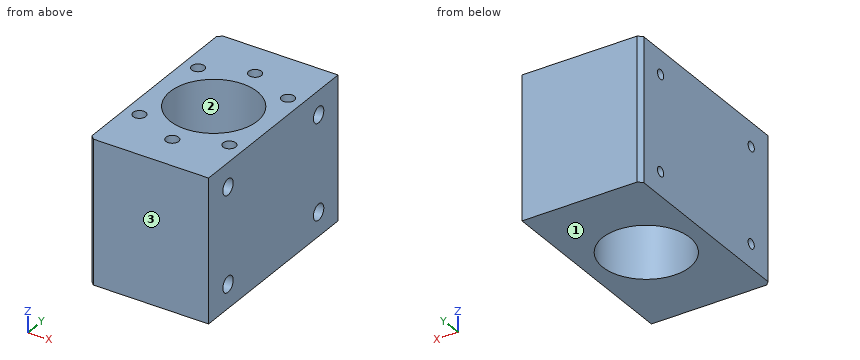
```python
from build123d import *

# Parameters (mm, degrees)
SKETCH_4_R          = 11
EXTRUDE_2_DEPTH     = 36
SKETCH_5_R          = 1.6
CUT_EXTRUDE_2_DEPTH = 10
SKETCH_6_R          = 2
CUT_EXTRUDE_3_DEPTH = 10
SKETCH_9_R          = 1.2
CUT_EXTRUDE_5_DEPTH = 5


with BuildPart() as part:
    # 草图4 → 凸台-拉伸2 (new body)
    with BuildSketch(Plane.XY):
        Polygon((15, 25), (-14, 25), (-15, 24), (-15, -24), (-14, -25), (15, -25), align=None)
        Circle(SKETCH_4_R, mode=Mode.SUBTRACT)
    extrude(amount=EXTRUDE_2_DEPTH)

    # 草图5 → 切除-拉伸2 (cut)
    with BuildSketch(Plane.XY.offset(36)):
        with Locations((0, 16)):
            Circle(SKETCH_5_R)
        with Locations((11.313708499, 11.313708499)):
            Circle(SKETCH_5_R)
        with Locations((11.313708499, -11.313708499)):
            Circle(SKETCH_5_R)
        with Locations((0, -16)):
            Circle(SKETCH_5_R)
        with Locations((-11.313708499, -11.313708499)):
            Circle(SKETCH_5_R)
        with Locations((-11.313708499, 11.313708499)):
            Circle(SKETCH_5_R)
    extrude(amount=-CUT_EXTRUDE_2_DEPTH, mode=Mode.SUBTRACT)

    # 草图6 → 切除-拉伸3 (cut)
    with BuildSketch(Plane(origin=(15, 0, 0), x_dir=(0, 0, -1), z_dir=(1, 0, 0))):
        with Locations((-6, 17.5)):
            Circle(SKETCH_6_R)
        with Locations((-30, 17.5)):
            Circle(SKETCH_6_R)
        with Locations((-30, -17.5)):
            Circle(SKETCH_6_R)
        with Locations((-6, -17.5)):
            Circle(SKETCH_6_R)
    extrude(amount=-CUT_EXTRUDE_3_DEPTH, mode=Mode.SUBTRACT)

    # 草图9 → 切除-拉伸5 (cut)
    with BuildSketch(Plane.ZY.offset(15)):
        with Locations((6, 17.5)):
            Circle(SKETCH_9_R)
        with Locations((30, 17.5)):
            Circle(SKETCH_9_R)
        with Locations((6, -17.5)):
            Circle(SKETCH_9_R)
        with Locations((30, -17.5)):
            Circle(SKETCH_9_R)
    extrude(amount=-CUT_EXTRUDE_5_DEPTH, mode=Mode.SUBTRACT)


solid = part.part
```
Input: part model. Units: mm. Frame: model coordinates. Face numbers are marked on the shaded views. Give positions to 0.01 mm unless a question says otherwise; leave off trailing zeros. Loops run counter-clockwise (first coordinate to the right, second up) from the corner with the lowest first, then second, coordinate; pieces in that order, holes last.
1) Line query: L1, parallel to Y at x = 13, z = 30; L2, parallel to Y at x = -12.9, z = 6; L3, parallel to Y at x = 0, z = 29.5. Output: solid intervals per line, ascending.
A:
L1: y = -25 to -19.5, -15.5 to 15.5, 19.5 to 25
L2: y = -25 to -18.7, -16.3 to 16.3, 18.7 to 25
L3: y = -25 to -17.6, -14.4 to -11, 11 to 14.4, 17.6 to 25
2) Mould query, pull axis Y, two halves, no side actions, for the marked faces 1, 2 and 3. Classes: released by +Y, released by -Y, zero draft, split by the parting line, or undercut.
A:
face 1: zero draft
face 2: undercut
face 3: released by -Y
3) Section query D-D on z = 6. Return the cut outline in (x, y), and give its area (3 significant figures).
A:
outline: (-15, -24) - (-14, -25) - (15, -25) - (15, -19.5) - (5, -19.5) - (5, -15.5) - (15, -15.5) - (15, 15.5) - (5, 15.5) - (5, 19.5) - (15, 19.5) - (15, 25) - (-14, 25) - (-15, 24) - (-15, 18.7) - (-10, 18.7) - (-10, 16.3) - (-15, 16.3) - (-15, -16.3) - (-10, -16.3) - (-10, -18.7) - (-15, -18.7) - close; hole circle Ø22 at (0, 0)
area: 1,010 mm2
4) Section query A-A on y = 0. Return the cut outline in (x, z), and give its area (3 significant figures).
A:
outline: (-15, 0) - (-11, 0) - (-11, 36) - (-15, 36) - close; (11, 0) - (15, 0) - (15, 36) - (11, 36) - close
area: 288 mm2
5) Section query B-B on z = 13. Return the cut outline in (x, y), and give its area (3 significant figures).
A:
outline: (-15, -24) - (-14, -25) - (15, -25) - (15, 25) - (-14, 25) - (-15, 24) - close; hole circle Ø22 at (0, 0)
area: 1,120 mm2
6) Contact query for flat-ended pins moving along their axis: pin 1 (1.9 mm diameter, centred on x = -11.31, y = -11.31, fed in from +Z); pin 2 (1.9 mm diameter, centred on y = -17.5, z = 6, fed in from -X); pin 3 (13 mm diameter, centred on x = 0, y = 0, fed in from -Z); pin 4 (1.9 mm diameter, centred on y = 17.5, z = 6, fed in from +X). Output: stop coordinate, or through.
A:
pin 1: stops at z = 26
pin 2: stops at x = -10
pin 3: passes through
pin 4: stops at x = 5
7) Section query C-C on x = 0. Return the cut outline in (y, z).
A:
outline: (-25, 0) - (-11, 0) - (-11, 36) - (-14.4, 36) - (-14.4, 26) - (-17.6, 26) - (-17.6, 36) - (-25, 36) - close; (11, 0) - (25, 0) - (25, 36) - (17.6, 36) - (17.6, 26) - (14.4, 26) - (14.4, 36) - (11, 36) - close
